from build123d import *

# Parameters (mm, degrees)
SKETCH1_W               = 312
SKETCH1_H               = 230
BOSS_EXTRUDE1_DEPTH     = 5
SKETCH2_W               = 4
SKETCH2_H               = 230
BOSS_EXTRUDE2_DEPTH     = 40
SKETCH3_R               = 50
CUT_EXTRUDE1_DEPTH      = 198.89138435
CUT_EXTRUDE2_DEPTH      = 198.89138435
CUT_EXTRUDE2_DEPTH_BACK = 198.89138435
SKETCH4_W               = 312
SKETCH4_H               = 10
SKETCH5_W               = 24.234530733
SKETCH5_H               = 45
CUT_EXTRUDE3_DEPTH      = 336.550294293


with BuildPart() as part:
    # Sketch1 → Boss-Extrude1 (new body)
    with BuildSketch(Plane(origin=(0, 0, 0), x_dir=(1, 0, 0), z_dir=(0, 1, 0))):
        Rectangle(SKETCH1_W, SKETCH1_H)
    extrude(amount=BOSS_EXTRUDE1_DEPTH)

    # Sketch2 → Boss-Extrude2 (add)
    with BuildSketch(Plane(origin=(0, 5, 0), x_dir=(1, 0, 0), z_dir=(0, 1, 0))):
        with Locations((-154, 0)):
            Rectangle(SKETCH2_W, SKETCH2_H)
        with Locations((154, 0)):
            Rectangle(SKETCH2_W, SKETCH2_H)
    extrude(amount=BOSS_EXTRUDE2_DEPTH)

    # Sketch3 → Cut-Extrude1 (cut, through all)
    with BuildSketch(Plane(origin=(0, 5, 0), x_dir=(1, 0, 0), z_dir=(0, 1, 0))):
        with Locations(Location((0, 0, 0), (0, 0, 270))):
            Circle(SKETCH3_R)
    extrude(amount=-CUT_EXTRUDE1_DEPTH, mode=Mode.SUBTRACT)

    # Sketch4 → Cut-Extrude2 (cut, two sides: drawn at the far end of the back side and taken through both)
    with BuildSketch(Plane(origin=(0, 5, 0), x_dir=(1, 0, 0), z_dir=(0, 1, 0)).offset(-CUT_EXTRUDE2_DEPTH_BACK)):
        with Locations((0, 110)):
            Rectangle(SKETCH4_W, SKETCH4_H)
    extrude(amount=CUT_EXTRUDE2_DEPTH + CUT_EXTRUDE2_DEPTH_BACK, mode=Mode.SUBTRACT)

    # Sketch5 → Cut-Extrude3 (cut, through all)
    with BuildSketch(Plane(origin=(156, 0, 0), x_dir=(0, 0, -1), z_dir=(1, 0, 0))):
        with Locations((-102.882734634, 22.5)):
            Rectangle(SKETCH5_W, SKETCH5_H)
    extrude(amount=-CUT_EXTRUDE3_DEPTH, mode=Mode.SUBTRACT)


solid = part.part
Read the model definition and answer for the solid it produces. Units are mm, in the model's axes. A direction names the side the tool comes from. Round coordinates to 2 decimals unless told otherwise and drop trailing zeros. Order: outer loops, then holes, each group sorted by start corner. A loop starts at its lowest first (then second) coordinate and runs counter-clockwise, first axis right, second up.
1) The part is cut by section B-B on x = 0. Write down the section's boundary in (y, z).
2) The part is cut by section D-D on x = 89.5. Write down the section's boundary in (y, z), plus the area to 3 significant figures.
3) The part is cut by section A-A on y = 14. Write down the section's boundary in (x, z).
4) The mould has two halves that part along X. Classify faces 1 (the face through (-1, 2, -105)), 2 (the face through (-152, 25, -6)), 3 (the face through (-156, 22, -6)): released by +X, released by -X, zero draft, split by the parting line, or undercut.
5) The part is cut by section C-C on z = 0. Write down the section's boundary in (x, y).
6) For faces 4 (the face through (15.02, 2.54, 47.69)), 5 (the face through (-2, 5, -52)), determine the directions among +Z, -Z, +X, -X, +Y, -Y from which every point of the face is accessible in a straight line to the end or side of a thin tool.
7) Straight lines are drawn through the part: L1, parallel to X at y = 23, z = -81; L2, parallel to X at y = 1, z = 0; L3, parallel to Y at x = 135.5, z = 29. For each, find the intervals that lie inside material, in ascending order.
Resolved:
1. outline: (0, -105) - (5, -105) - (5, -50) - (0, -50) - close; (0, 50) - (5, 50) - (5, 90.77) - (0, 90.77) - close
2. outline: (0, -105) - (5, -105) - (5, 90.77) - (0, 90.77) - close
2. area: 979 mm2
3. outline: (-156, -105) - (-152, -105) - (-152, 90.77) - (-156, 90.77) - close; (152, -105) - (156, -105) - (156, 90.77) - (152, 90.77) - close
4. face 1: zero draft
4. face 2: undercut
4. face 3: released by -X
5. outline: (-156, 0) - (-50, 0) - (-50, 5) - (-152, 5) - (-152, 45) - (-156, 45) - close; (50, 0) - (156, 0) - (156, 45) - (152, 45) - (152, 5) - (50, 5) - close
6. face 4: +Y, -Y
6. face 5: +Z, -Z, +Y
7. L1: x = -156 to -152, 152 to 156
7. L2: x = -156 to -50, 50 to 156
7. L3: y = 0 to 5
